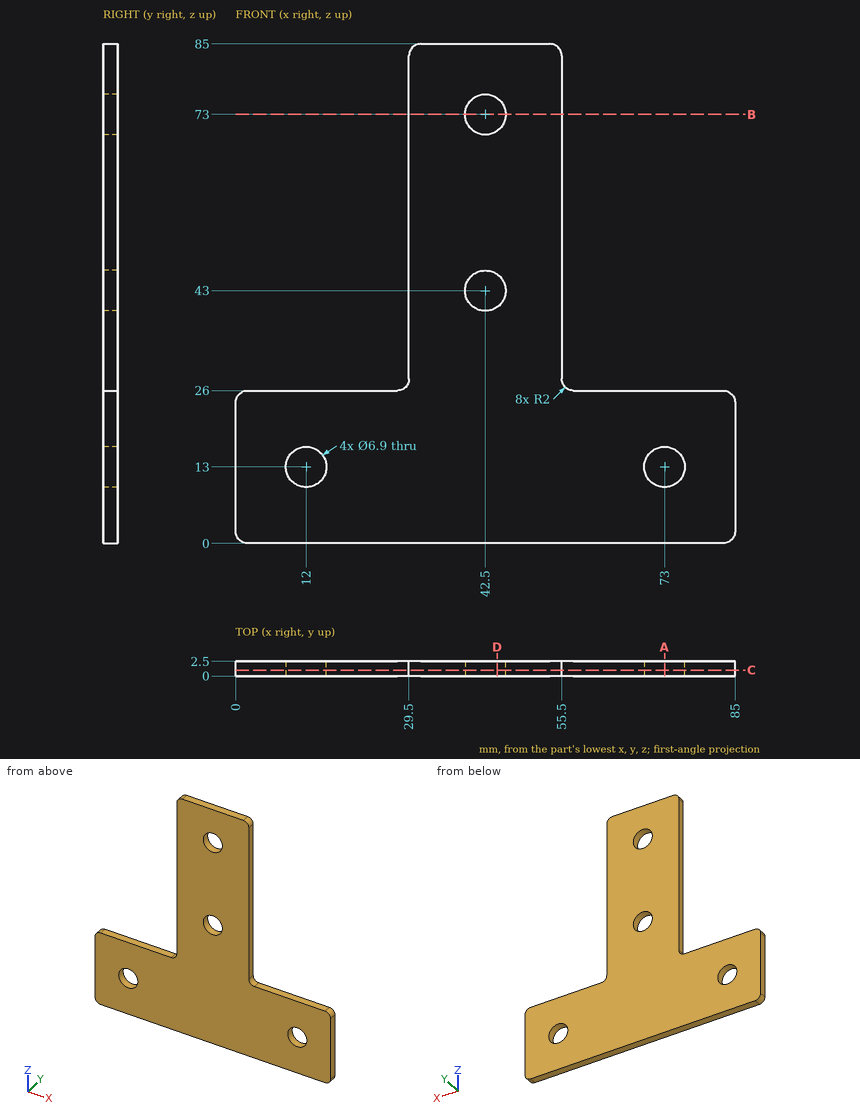
Geometry check sheet. Reference: drawing and pictorial views, mm from the part's lowest x, y, z. Round coordinates to 2 decimals unless told otherwise and drop trailing zeros. Write each loop counter-clockwise with the first axis right and the second up, starting at its lowest first coordinate (ties: lowest second). Pieces come first, ordered by that corner, then holes.
(1) Section check B-B (z = 73). Enter the section's corners in (x, y), plus the area to 4 significant figures.
Returned:
outline: (29.5, 0) - (39.05, 0) - (39.05, 2.5) - (29.5, 2.5) - close; (45.95, 0) - (55.5, 0) - (55.5, 2.5) - (45.95, 2.5) - close
area: 47.75 mm2
(2) Depth check by flat-ended pin: pin 1 Ø4 at (x, z) = (12, 13) entering from -Y; pin 2 Ø0.8 at (x, y) = (67.5, 1) entering from +Z; pin 3 Ø0.8 at (y, z) = (1, 62.5) entering from +X. Enter the tip coordinate at first touch or a pass-through.
Returned:
pin 1: passes through
pin 2: stops at z = 26
pin 3: stops at x = 55.5
(3) Section check A-A (x = 73). Enter the section's corners in (y, z), plus the area to 4 significant figures.
Returned:
outline: (0, 0) - (2.5, 0) - (2.5, 9.55) - (0, 9.55) - close; (0, 16.45) - (2.5, 16.45) - (2.5, 26) - (0, 26) - close
area: 47.75 mm2
(4) Section check D-D (x = 44.5). Enter the section's corners in (y, z), plus the area to 3 significant figures.
Returned:
outline: (0, 0) - (2.5, 0) - (2.5, 40.19) - (0, 40.19) - close; (0, 45.81) - (2.5, 45.81) - (2.5, 70.19) - (0, 70.19) - close; (0, 75.81) - (2.5, 75.81) - (2.5, 85) - (0, 85) - close
area: 184 mm2
(5) Material ranges on line 1 (Z direction, x = 42.5, y = 0.8); line 2 (Z direction, x = 73, y = 1.45); line 3 (X direction, y = 1.4, z = 13), recorded low to high.
Returned:
line 1: z = 0 to 39.55, 46.45 to 69.55, 76.45 to 85
line 2: z = 0 to 9.55, 16.45 to 26
line 3: x = 0 to 8.55, 15.45 to 69.55, 76.45 to 85
(6) Section check C-C (y = 1). Enter the section's corners in (x, z).
Returned:
outline: (0, 2) arc R2 ccw to (2, 0) - (83, 0) arc R2 ccw to (85, 2) - (85, 24) arc R2 ccw to (83, 26) - (57.5, 26) arc R2 cw to (55.5, 28) - (55.5, 83) arc R2 ccw to (53.5, 85) - (31.5, 85) arc R2 ccw to (29.5, 83) - (29.5, 28) arc R2 cw to (27.5, 26) - (2, 26) arc R2 ccw to (0, 24) - close; hole circle Ø6.9 at (12, 13); hole circle Ø6.9 at (42.5, 43); hole circle Ø6.9 at (42.5, 73); hole circle Ø6.9 at (73, 13)
